Autodesk Inventor part; units mm, degrees
ref_plane "YZ Plane" through (0, 0, 0) normal (1, 0, 0) x (0, 1, 0)
ref_plane "XZ Plane" through (0, 0, 0) normal (0, 1, 0) x (-1, 0, 0)
ref_plane "XY Plane" through (0, 0, 0) normal (0, 0, 1) x (1, 0, 0)
sketch "Sketch1" plane through (0, 0, 0) normal (0, 1, 0) x (-1, 0, 0)
  line L0 (0, 0) -> (73, 0)
  line L1 (73, 0) -> (73, -148)
  line L2 (73, -148) -> (0, -148)
  line L3 (0, -148) -> (0, 0)
  dimension "d0" = 73
  dimension "d1" = 148
extrude "Extrusion1" add sketch "Sketch1" against normal blind 4
sketch "Sketch2" plane through (0, 0, 0) normal (0, 1, 0) x (1, 0, 0)
  line L0 (-73, 148) -> (0, 148)
  line L1 (0, 148) -> (0, 0)
  line L2 (0, 148) -> (0, 0)
  line L3 (0, 0) -> (-73, 0)
  line L4 (0, 0) -> (-73, 0)
  line L5 (-73, 0) -> (-73, 148)
  line L6 (0, 148) -> (0, 144) construction
  line L7 (0, 148) -> (0, 0) construction
  line L8 (0, 144) -> (-4, 144) construction
  line L9 (-4, 144) -> (-69, 144)
  line L10 (-69, 144) -> (-69, 4)
  line L11 (-69, 4) -> (-4, 4)
  line L12 (-4, 4) -> (-4, 144)
  dimension "d4" = 4
  dimension "d5" = 4
  dimension "d6" = 90
  dimension "d7" = 65
  dimension "d8" = 140
extrude "Extrusion2" add sketch "Sketch2" along normal blind 22
sketch "Sketch3" plane through (0, 22, 0) normal (0, 1, 0) x (1, 0, 0)
  line L0 (-4, 4) -> (-69, 4)
  line L1 (-4, 4) -> (-2.1, 4) construction
  line L2 (-2.1, 4) -> (-2.1, 2.1) construction
  line L3 (-2.1, 2.1) -> (-71.1, 2.1)
  line L4 (-73, 148) -> (-73, 0)
  line L5 (-71.1, 2.1) -> (-71.1, 146.1)
  line L6 (-71.1, 146.1) -> (-2.1, 146.1)
  line L7 (-2.1, 146.1) -> (-2.1, 2.1)
  line L8 (-73, 0) -> (0, 0)
  line L9 (0, 148) -> (-73, 148)
  line L10 (-73, 0) -> (-73, 148)
  line L11 (-73, 148) -> (0, 148)
  line L12 (0, 148) -> (0, 0)
  point P0 (-4, 144)
  point P1 (-69, 144)
  dimension "d11" = 1.9
  dimension "d12" = 1.9
  dimension "d13" = 69
  dimension "d14" = 144
  dimension "d15" = 69
extrude "Extrusion3" cut sketch "Sketch3" against normal blind 4
sketch "Sketch4" plane through (0, 0, 0) normal (0, 1, 0) x (1, 0, 0)
  line L0 (-69, 4) -> (-69, 144)
  line L1 (-69, 144) -> (-63, 144)
  line L2 (-63, 144) -> (-63, 138)
  line L3 (-63, 138) -> (-69, 138)
  line L4 (-69, 138) -> (-69, 144)
  point P0 (0, 0)
  dimension "d18" = 6
  dimension "d19" = 6
extrude "Extrusion4" add sketch "Sketch4" along normal blind 15
sketch "Sketch5" plane through (0, 22, 0) normal (0, 1, 0) x (1, 0, 0)
  line L0 (-69, 138) -> (-63, 138) construction
  line L1 (-63, 138) -> (-66, 138) construction
  line L2 (-63, 138) -> (-60, 138) construction
  line L3 (-66, 138) -> (-66, 141) construction
  circle A0 centre (-66, 141) radius 2
  point P0 (0, 0)
  dimension "d22" = 3
  dimension "d23" = 180
  dimension "d24" = 3
  dimension "d25" = 4
extrude "Extrusion5" cut sketch "Sketch5" against normal blind 20
sketch "Sketch6" plane through (0, -4, 0) normal (0, -1, 0) x (1, 0, 0)
  line L0 (-73, 0) -> (-73, -148) construction
  line L1 (-73, -148) -> (-73, -141) construction
  line L2 (-73, -141) -> (-66, -141) construction
  circle A0 centre (-66, -141) radius 4
  point P0 (0, 0)
  dimension "d28" = 7
  dimension "d41" = 7
  dimension "d42" = 8
extrude "Extrusion6" cut sketch "Sketch6" against normal blind 4
pattern_linear "Rectangular Pattern1" count 2 spacing 59 along (1, 0, 0) count 2 spacing 134 along (0, 0, 1) of "Extrusion4", "Extrusion5", "Extrusion6"
sketch "Sketch7" plane through (0, 0, 0) normal (0, 1, 0) x (1, 0, 0)
  line L0 (-69, 138) -> (-63, 138)
  line L1 (-69, 138) -> (-63, 138)
  line L2 (-10, 144) -> (-63, 144)
  line L3 (-63, 138) -> (-63, 144)
  line L4 (-63, 144) -> (-61.4, 144)
  line L5 (-69, 138) -> (-69, 136.4)
  line L6 (-69, 138) -> (-69, 10)
  line L7 (-69, 136.4) -> (-61.4, 136.4)
  line L8 (-61.4, 136.4) -> (-61.4, 144)
  point P0 (0, 0)
  dimension "d43" = 1.6
  dimension "d44" = 1.6
extrude "Extrusion7" add sketch "Sketch7" along normal blind 1.2
sketch "Sketch8" plane through (0, 0, 0) normal (0, 1, 0) x (1, 0, 0)
  line L0 (-10, 4) -> (-10, 4.3542)
  line L1 (-10, 4) -> (-11.6, 4)
  line L2 (-4, 4) -> (-69, 4)
  line L3 (-4, 10) -> (-10, 10)
  line L4 (-10, 4) -> (-10, 10)
  line L5 (-10, 10) -> (-4, 10)
  line L6 (-4, 10) -> (-4, 11.6)
  line L7 (-4, 11.6) -> (-11.6, 11.6)
  line L8 (-11.6, 11.6) -> (-11.6, 4)
  line L9 (-11.6, 11.6) -> (-69, 11.6) construction
  line L10 (-69, 136.4) -> (-69, 10)
  line L11 (-69, 10) -> (-69, 11.6)
  line L12 (-69, 10) -> (-63, 10)
  line L13 (-63, 10) -> (-63, 4)
  line L14 (-63, 4) -> (-61.4, 4)
  line L15 (-63, 4) -> (-10, 4)
  line L16 (-61.4, 4) -> (-61.4, 11.6)
  line L17 (-69, 11.6) -> (-61.4, 11.6)
  line L18 (-9.6458, 138) -> (-10, 138)
  line L19 (-4, 138) -> (-2.4, 138) construction
  line L20 (-10, 144) -> (-61.4, 144)
  line L21 (-10, 138) -> (-10, 144)
  line L22 (-10, 144) -> (-11.6, 144)
  line L23 (-10, 138) -> (-4, 138)
  line L24 (-4, 138) -> (-4, 136.4)
  line L25 (-4, 10) -> (-4, 138)
  line L26 (-4, 136.4) -> (-11.6, 136.4)
  line L27 (-11.6, 136.4) -> (-11.6, 144)
  point P0 (0, 0)
  dimension "d47" = 1.6
  dimension "d48" = 1.6
  dimension "d49" = 1.6
  dimension "d55" = 7.6
  dimension "d56" = 7.6
  dimension "d57" = 1.6
  dimension "d58" = 1.6
  dimension "d59" = 90
extrude "Extrusion8" add sketch "Sketch8" along normal blind 1.2
sketch "Sketch9" plane through (-69, 15, -10) normal (0, 1, 0) x (1, 0, 0)
  line L0 (6, -6) -> (6, 0)
  line L1 (0, -6) -> (0, 134)
  line L2 (6, 0) -> (0, 0)
  line L3 (0, 0) -> (0, -6)
  line L4 (0, -6) -> (6, -6)
  line L5 (6, -6) -> (6, 0)
  line L6 (65, 134) -> (65, -6)
  line L7 (65, 1.6) -> (65, -6)
  line L8 (65, -6) -> (57.4, -6)
  line L9 (59, 134) -> (59, 128)
  line L10 (65, 134) -> (59, 134)
  line L11 (59, 134) -> (59, 128)
  line L12 (59, 128) -> (65, 128)
  line L13 (65, 128) -> (65, 134)
  line L14 (65, -6) -> (59, -6)
  line L15 (65, -6) -> (59, -6)
  line L16 (59, -6) -> (59, 0)
  line L17 (59, 0) -> (65, 0)
  line L18 (65, 0) -> (65, -6)
  line L19 (6, 128) -> (6, 134)
  line L20 (0, 134) -> (6, 134)
  line L21 (6, 128) -> (0, 128)
  line L22 (0, 128) -> (0, 134)
  line L23 (0, 134) -> (6, 134)
  line L24 (6, 134) -> (6, 128)
  point P0 (69, -10)
  point P1 (57.4, 1.6)
extrude "Extrusion9" add sketch "Sketch9" along normal blind 6
sketch "Sketch10" plane through (-66, 0, -7) normal (0, -1, 0) x (1, 0, 0)
  circle A0 centre (0, 0) radius 2.05
  circle A1 centre (59, 0) radius 2
  circle A2 centre (59, 0) radius 2.05
  circle A3 centre (0, -134) radius 2
  circle A4 centre (0, -134) radius 2.05
  circle A5 centre (59, -134) radius 2.05
  point P0 (66, 7)
  dimension "d64" = 4.1
  dimension "d65" = 4.1
  dimension "d66" = 4.1
  dimension "d67" = 4.1
extrude "Extrusion10" cut sketch "Sketch10" against normal blind 200 contours A0 | A1 | A3 | A5
sketch "Sketch11" plane through (-7, 0, -7) normal (0, -1, 0) x (1, 0, 0)
  circle A0 centre (0, 0) radius 2.05
  point P0 (7, 7)
  dimension "d70" = 4.1
extrude "Extrusion11" cut sketch "Sketch11" against normal blind 100
sketch "Sketch12" plane through (-66, 0, -141) normal (0, -1, 0) x (1, 0, 0)
  circle A0 centre (0, 0) radius 2.05
  point P0 (66, 141)
  dimension "d73" = 4.1
extrude "Extrusion12" cut sketch "Sketch12" against normal blind 100
chamfer "Chamfer1" distance 2 angle 45 8 edges at (-36.5, -4, 0) (-73, 7, 0) (-73, -4, -74) (0, 7, 0) (0, -4, -74) (0, 7, -148) (-36.5, -4, -148) (-73, 7, -148)
properties part number "mangOH bottom"
Could you check a few things on this model? Use its own coordinates, in mm. A direction names the side the tool comes from. Give positions to 0.01 mm unless a question says otherwise; leave off trailing zeros. Write each loop counter-clockwise with the first axis right and the second up, starting at its lowest first coordinate (ties: lowest second). Pieces come first, ordered by that corner, then holes. Notation, with made-up numbers: (49, 79) -> (101, 79) arc R10 cw to (101, 97) -> close; hole circle Ø10 at (55.5, 70.5). An arc over 180 degrees is marked (long way). Answer as a JSON object with one key per item and string values.
Q1. Which directions (+Z, -Z, +X, -X, +Y, -Y) give clear straight access to the entire face, cutting with the end or side of a thin tool? Please do faces 4 (the cylindrical face through (-66.267, 10.353, -138.967)), 5 (the flat face through (-66, 11, -138)), 6 (the cylindrical face through (-10.2, -2, -9.4)).
Taken from the geometry:
{"face 4": "+Y, -Y", "face 5": "+Y", "face 6": "-Y"}
Q2. Suppose I cut it at C-C on z = -78.5. Write out the boundary of the cut face in (x, y), then the cut area to 3 significant figures.
Taken from the geometry:
{"outline": "(-73, -2) -> (-71, -4) -> (-2, -4) -> (0, -2) -> (0, 18) -> (-2.1, 18) -> (-2.1, 22) -> (-4, 22) -> (-4, 0) -> (-69, 0) -> (-69, 22) -> (-71.1, 22) -> (-71.1, 18) -> (-73, 18) -> close", "area": "448 mm²"}
Q3. Suppose I cut it at B-B on x = -55. Write out the boundary of the cut face in (y, z).
Taken from the geometry:
{"outline": "(-4, -146) -> (-2, -148) -> (18, -148) -> (18, -146.1) -> (22, -146.1) -> (22, -144) -> (0, -144) -> (0, -4) -> (22, -4) -> (22, -2.1) -> (18, -2.1) -> (18, 0) -> (-2, 0) -> (-4, -2) -> close"}
Q4. We'd pull the mould along Z, two halves only. Please class faces 1 (the flat face through (-36, 8, 0)), 2 (the flat face through (-2.1, 20, -75)), 3 (the cylindrical face through (-7.521, -2.028, -137.034)): released by +Z, released by -Z, zero draft, split by the parting line, or undercut.
Taken from the geometry:
{"face 1": "released by +Z", "face 2": "zero draft", "face 3": "undercut"}
Q5. Suppose I cut it at D-D on z = -141. Count the separate pieces of the cut face and the enclosed holes in it, then the cut area to 3 significant figures.
Taken from the geometry:
{"separate pieces": "3", "enclosed holes": "0", "area": "468 mm²"}
Q6. Suppose I cut it at A-A on y = 13.75. Write out the boundary of the cut face in (x, z), then the cut area to 3 significant figures.
Taken from the geometry:
{"outline": "(-73, -146) -> (-71, -148) -> (-2, -148) -> (0, -146) -> (0, -2) -> (-2, 0) -> (-71, 0) -> (-73, -2) -> close; hole (-69, -138) -> (-63, -138) -> (-63, -144) -> (-10, -144) -> (-10, -138) -> (-4, -138) -> (-4, -10) -> (-10, -10) -> (-10, -4) -> (-63, -4) -> (-63, -10) -> (-69, -10) -> close; hole circle Ø4.1 at (-66, -141); hole circle Ø4.1 at (-66, -7); hole circle Ø4.1 at (-7, -141); hole circle Ø4.1 at (-7, -7)", "area": "1,790 mm²"}
Q7. Please list where these lines run through material, in increasing order: L1, parallel to X at y = 9.25, z = -141; L2, parallel to X at y = -1.7, z = -141; L3, parallel to Z at x = -66, y = 5.5.
Taken from the geometry:
{"L1": "x = -73 to -68.05, -63.95 to -63, -10 to -9.05, -4.95 to 0", "L2": "x = -73 to -70, -62 to -11, -3 to 0", "L3": "z = -148 to -143.05, -138.95 to -138, -10 to -9.05, -4.95 to 0"}
Q8. Will these pins go through, and if not, where does the flat tip stop? pin 1 Ø1 at (x, z) = (-51.5, -55) entering from +Y; pin 2 Ø3.5 at (x, z) = (-7, -7) entering from +Y; pin 3 Ø5 at (x, z) = (-7, -8.5) entering from +Y.
Taken from the geometry:
{"pin 1": "stops at y = 0", "pin 2": "passes through", "pin 3": "stops at y = 21"}
